from build123d import *

# Parameters (mm, degrees)
SKETCH_1_W          = 41.47467615
SKETCH_1_H          = 18.100023376
EXTRUDE_1_DEPTH     = 2
CUT_EXTRUDE_1_REACH = 26.88
SKETCH_2_R          = 1.4
CUT_EXTRUDE_2_REACH = 26.88


with BuildPart() as part:
    # 草图1 → 凸台-拉伸1 (new body)
    with BuildSketch(Plane.XY):
        with Locations((0, 4.550011688)):
            Rectangle(SKETCH_1_W, SKETCH_1_H)
    extrude(amount=EXTRUDE_1_DEPTH)

    # 草图2 → 切除-拉伸1 (cut, up to next)
    with BuildSketch(Plane.XY.offset(2), mode=Mode.PRIVATE) as cut_extrude_1_sk1:
        with Locations((-18.383061341, -2.4)):
            Circle(SKETCH_2_R)
    cut_extrude_1_tool1 = extrude(cut_extrude_1_sk1.sketch, amount=-CUT_EXTRUDE_1_REACH, mode=Mode.PRIVATE) & part.part
    # 草图2 → 切除-拉伸1 (cut, up to next)
    with BuildSketch(Plane.XY.offset(2), mode=Mode.PRIVATE) as cut_extrude_1_sk2:
        with Locations(Location((18.383061341, -2.4, 0), (0, 0, 180))):
            Circle(SKETCH_2_R)
    cut_extrude_1_tool2 = extrude(cut_extrude_1_sk2.sketch, amount=-CUT_EXTRUDE_1_REACH, mode=Mode.PRIVATE) & part.part
    # 草图2 → 切除-拉伸1 (cut, up to next)
    with BuildSketch(Plane.XY.offset(2), mode=Mode.PRIVATE) as cut_extrude_1_sk3:
        with Locations((18.383061341, 11.500023376)):
            Circle(SKETCH_2_R)
    cut_extrude_1_tool3 = extrude(cut_extrude_1_sk3.sketch, amount=-CUT_EXTRUDE_1_REACH, mode=Mode.PRIVATE) & part.part
    # 草图2 → 切除-拉伸1 (cut, up to next)
    with BuildSketch(Plane.XY.offset(2), mode=Mode.PRIVATE) as cut_extrude_1_sk4:
        with Locations(Location((-18.383061341, 11.500023376, 0), (0, 0, 180))):
            Circle(SKETCH_2_R)
    cut_extrude_1_tool4 = extrude(cut_extrude_1_sk4.sketch, amount=-CUT_EXTRUDE_1_REACH, mode=Mode.PRIVATE) & part.part
    add(cut_extrude_1_tool1.solids().sort_by_distance((-18.383061, -2.4, 2))[0], mode=Mode.SUBTRACT)
    add(cut_extrude_1_tool2.solids().sort_by_distance((18.383061, -2.4, 2))[0], mode=Mode.SUBTRACT)
    add(cut_extrude_1_tool3.solids().sort_by_distance((18.383061, 11.500023, 2))[0], mode=Mode.SUBTRACT)
    add(cut_extrude_1_tool4.solids().sort_by_distance((-18.383061, 11.500023, 2))[0], mode=Mode.SUBTRACT)

    # 草图3 → 切除-拉伸2 (cut, up to next)
    with BuildSketch(Plane(origin=(0, 0, 0), x_dir=(-1, 0, 0), z_dir=(0, 0, -1)), mode=Mode.PRIVATE) as cut_extrude_2_sk1:
        Polygon((-20.737338075, 1.050011688), (-20.437338075, 1.050011688), (-20.237338075, 0.850011688), (-20.237338075, 0.250011688), (-20.437338075, 0.050011688), (-20.737338075, 0.050011688), align=None)
    cut_extrude_2_tool1 = extrude(cut_extrude_2_sk1.sketch, amount=-CUT_EXTRUDE_2_REACH, mode=Mode.PRIVATE) & part.part
    # 草图3 → 切除-拉伸2 (cut, up to next)
    with BuildSketch(Plane(origin=(0, 0, 0), x_dir=(-1, 0, 0), z_dir=(0, 0, -1)), mode=Mode.PRIVATE) as cut_extrude_2_sk2:
        Polygon((-20.737338075, 2.550011688), (-20.437338075, 2.550011688), (-20.237338075, 2.350011688), (-20.237338075, 1.750011688), (-20.437338075, 1.550011688), (-20.737338075, 1.550011688), align=None)
    cut_extrude_2_tool2 = extrude(cut_extrude_2_sk2.sketch, amount=-CUT_EXTRUDE_2_REACH, mode=Mode.PRIVATE) & part.part
    # 草图3 → 切除-拉伸2 (cut, up to next)
    with BuildSketch(Plane(origin=(0, 0, 0), x_dir=(-1, 0, 0), z_dir=(0, 0, -1)), mode=Mode.PRIVATE) as cut_extrude_2_sk3:
        Polygon((-20.737338075, 4.050011688), (-20.437338075, 4.050011688), (-20.237338075, 3.850011688), (-20.237338075, 3.250011688), (-20.437338075, 3.050011688), (-20.737338075, 3.050011688), align=None)
    cut_extrude_2_tool3 = extrude(cut_extrude_2_sk3.sketch, amount=-CUT_EXTRUDE_2_REACH, mode=Mode.PRIVATE) & part.part
    # 草图3 → 切除-拉伸2 (cut, up to next)
    with BuildSketch(Plane(origin=(0, 0, 0), x_dir=(-1, 0, 0), z_dir=(0, 0, -1)), mode=Mode.PRIVATE) as cut_extrude_2_sk4:
        Polygon((-20.737338075, 5.550011688), (-20.437338075, 5.550011688), (-20.237338075, 5.350011688), (-20.237338075, 4.750011688), (-20.437338075, 4.550011688), (-20.737338075, 4.550011688), align=None)
    cut_extrude_2_tool4 = extrude(cut_extrude_2_sk4.sketch, amount=-CUT_EXTRUDE_2_REACH, mode=Mode.PRIVATE) & part.part
    # 草图3 → 切除-拉伸2 (cut, up to next)
    with BuildSketch(Plane(origin=(0, 0, 0), x_dir=(-1, 0, 0), z_dir=(0, 0, -1)), mode=Mode.PRIVATE) as cut_extrude_2_sk5:
        Polygon((-20.737338075, 7.050011688), (-20.437338075, 7.050011688), (-20.237338075, 6.850011688), (-20.237338075, 6.250011688), (-20.437338075, 6.050011688), (-20.737338075, 6.050011688), align=None)
    cut_extrude_2_tool5 = extrude(cut_extrude_2_sk5.sketch, amount=-CUT_EXTRUDE_2_REACH, mode=Mode.PRIVATE) & part.part
    # 草图3 → 切除-拉伸2 (cut, up to next)
    with BuildSketch(Plane(origin=(0, 0, 0), x_dir=(-1, 0, 0), z_dir=(0, 0, -1)), mode=Mode.PRIVATE) as cut_extrude_2_sk6:
        Polygon((-20.737338075, 8.550011688), (-20.437338075, 8.550011688), (-20.237338075, 8.350011688), (-20.237338075, 7.750011688), (-20.437338075, 7.550011688), (-20.737338075, 7.550011688), align=None)
    cut_extrude_2_tool6 = extrude(cut_extrude_2_sk6.sketch, amount=-CUT_EXTRUDE_2_REACH, mode=Mode.PRIVATE) & part.part
    # 草图3 → 切除-拉伸2 (cut, up to next)
    with BuildSketch(Plane(origin=(0, 0, 0), x_dir=(-1, 0, 0), z_dir=(0, 0, -1)), mode=Mode.PRIVATE) as cut_extrude_2_sk7:
        Polygon((-20.737338075, 10.050011688), (-20.437338075, 10.050011688), (-20.237338075, 9.850011688), (-20.237338075, 9.250011688), (-20.437338075, 9.050011688), (-20.737338075, 9.050011688), align=None)
    cut_extrude_2_tool7 = extrude(cut_extrude_2_sk7.sketch, amount=-CUT_EXTRUDE_2_REACH, mode=Mode.PRIVATE) & part.part
    # 草图3 → 切除-拉伸2 (cut, up to next)
    with BuildSketch(Plane(origin=(0, 0, 0), x_dir=(-1, 0, 0), z_dir=(0, 0, -1)), mode=Mode.PRIVATE) as cut_extrude_2_sk8:
        Polygon((20.737338075, 3.050011688), (20.737338075, 4.050011688), (20.437338075, 4.050011688), (20.237338075, 3.850011688), (20.237338075, 3.250011688), (20.437338075, 3.050011688), align=None)
    cut_extrude_2_tool8 = extrude(cut_extrude_2_sk8.sketch, amount=-CUT_EXTRUDE_2_REACH, mode=Mode.PRIVATE) & part.part
    # 草图3 → 切除-拉伸2 (cut, up to next)
    with BuildSketch(Plane(origin=(0, 0, 0), x_dir=(-1, 0, 0), z_dir=(0, 0, -1)), mode=Mode.PRIVATE) as cut_extrude_2_sk9:
        Polygon((20.737338075, 1.550011688), (20.737338075, 2.550011688), (20.437338075, 2.550011688), (20.237338075, 2.350011688), (20.237338075, 1.750011688), (20.437338075, 1.550011688), align=None)
    cut_extrude_2_tool9 = extrude(cut_extrude_2_sk9.sketch, amount=-CUT_EXTRUDE_2_REACH, mode=Mode.PRIVATE) & part.part
    # 草图3 → 切除-拉伸2 (cut, up to next)
    with BuildSketch(Plane(origin=(0, 0, 0), x_dir=(-1, 0, 0), z_dir=(0, 0, -1)), mode=Mode.PRIVATE) as cut_extrude_2_sk10:
        Polygon((20.737338075, 4.550011688), (20.737338075, 5.550011688), (20.437338075, 5.550011688), (20.237338075, 5.350011688), (20.237338075, 4.750011688), (20.437338075, 4.550011688), align=None)
    cut_extrude_2_tool10 = extrude(cut_extrude_2_sk10.sketch, amount=-CUT_EXTRUDE_2_REACH, mode=Mode.PRIVATE) & part.part
    # 草图3 → 切除-拉伸2 (cut, up to next)
    with BuildSketch(Plane(origin=(0, 0, 0), x_dir=(-1, 0, 0), z_dir=(0, 0, -1)), mode=Mode.PRIVATE) as cut_extrude_2_sk11:
        Polygon((20.737338075, 6.050011688), (20.737338075, 7.050011688), (20.437338075, 7.050011688), (20.237338075, 6.850011688), (20.237338075, 6.250011688), (20.437338075, 6.050011688), align=None)
    cut_extrude_2_tool11 = extrude(cut_extrude_2_sk11.sketch, amount=-CUT_EXTRUDE_2_REACH, mode=Mode.PRIVATE) & part.part
    # 草图3 → 切除-拉伸2 (cut, up to next)
    with BuildSketch(Plane(origin=(0, 0, 0), x_dir=(-1, 0, 0), z_dir=(0, 0, -1)), mode=Mode.PRIVATE) as cut_extrude_2_sk12:
        Polygon((20.737338075, 7.550011688), (20.737338075, 8.550011688), (20.437338075, 8.550011688), (20.237338075, 8.350011688), (20.237338075, 7.750011688), (20.437338075, 7.550011688), align=None)
    cut_extrude_2_tool12 = extrude(cut_extrude_2_sk12.sketch, amount=-CUT_EXTRUDE_2_REACH, mode=Mode.PRIVATE) & part.part
    # 草图3 → 切除-拉伸2 (cut, up to next)
    with BuildSketch(Plane(origin=(0, 0, 0), x_dir=(-1, 0, 0), z_dir=(0, 0, -1)), mode=Mode.PRIVATE) as cut_extrude_2_sk13:
        Polygon((20.737338075, 9.050011688), (20.737338075, 10.050011688), (20.437338075, 10.050011688), (20.237338075, 9.850011688), (20.237338075, 9.250011688), (20.437338075, 9.050011688), align=None)
    cut_extrude_2_tool13 = extrude(cut_extrude_2_sk13.sketch, amount=-CUT_EXTRUDE_2_REACH, mode=Mode.PRIVATE) & part.part
    # 草图3 → 切除-拉伸2 (cut, up to next)
    with BuildSketch(Plane(origin=(0, 0, 0), x_dir=(-1, 0, 0), z_dir=(0, 0, -1)), mode=Mode.PRIVATE) as cut_extrude_2_sk14:
        Polygon((20.737338075, 0.050011688), (20.737338075, 1.050011688), (20.437338075, 1.050011688), (20.237338075, 0.850011688), (20.237338075, 0.250011688), (20.437338075, 0.050011688), align=None)
    cut_extrude_2_tool14 = extrude(cut_extrude_2_sk14.sketch, amount=-CUT_EXTRUDE_2_REACH, mode=Mode.PRIVATE) & part.part
    add(cut_extrude_2_tool1.solids().sort_by_distance((20.50328, 0.550012, 0))[0], mode=Mode.SUBTRACT)
    add(cut_extrude_2_tool2.solids().sort_by_distance((20.50328, 2.050012, 0))[0], mode=Mode.SUBTRACT)
    add(cut_extrude_2_tool3.solids().sort_by_distance((20.50328, 3.550012, 0))[0], mode=Mode.SUBTRACT)
    add(cut_extrude_2_tool4.solids().sort_by_distance((20.50328, 5.050012, 0))[0], mode=Mode.SUBTRACT)
    add(cut_extrude_2_tool5.solids().sort_by_distance((20.50328, 6.550012, 0))[0], mode=Mode.SUBTRACT)
    add(cut_extrude_2_tool6.solids().sort_by_distance((20.50328, 8.050012, 0))[0], mode=Mode.SUBTRACT)
    add(cut_extrude_2_tool7.solids().sort_by_distance((20.50328, 9.550012, 0))[0], mode=Mode.SUBTRACT)
    add(cut_extrude_2_tool8.solids().sort_by_distance((-20.50328, 3.550012, 0))[0], mode=Mode.SUBTRACT)
    add(cut_extrude_2_tool9.solids().sort_by_distance((-20.50328, 2.050012, 0))[0], mode=Mode.SUBTRACT)
    add(cut_extrude_2_tool10.solids().sort_by_distance((-20.50328, 5.050012, 0))[0], mode=Mode.SUBTRACT)
    add(cut_extrude_2_tool11.solids().sort_by_distance((-20.50328, 6.550012, 0))[0], mode=Mode.SUBTRACT)
    add(cut_extrude_2_tool12.solids().sort_by_distance((-20.50328, 8.050012, 0))[0], mode=Mode.SUBTRACT)
    add(cut_extrude_2_tool13.solids().sort_by_distance((-20.50328, 9.550012, 0))[0], mode=Mode.SUBTRACT)
    add(cut_extrude_2_tool14.solids().sort_by_distance((-20.50328, 0.550012, 0))[0], mode=Mode.SUBTRACT)


solid = part.part
CAD build for the part. Positions are in the model's coordinates, mm. Give positions to 0.01 mm unless a question says otherwise; leave off trailing zeros. Write each loop counter-clockwise with the first axis right and the second up, starting at its lowest first coordinate (ties: lowest second). Pieces come first, ordered by that corner, then holes. Notation, with made-up numbers: (81.25, -28.5) - (106.25, -28.5) arc R17 cw to (106.25, -6.5) - close; hole circle Ø1 at (55, 12). An arc over 180 degrees is marked (long way). Answer as CSV lines item,"result".
Q1. Pull direction Y, two halves, no side cores. Call faces 1 (the face through (0, 13.6, 1)), 2 (the face through (-19.78, -2.34, 1.01)), 3 (the face through (0, -4.5, 1)), 4 (the face through (0, 5, 0)): released by +Y, released by -Y, zero draft, split by the parting line, or undercut.
Result set:
face 1,"released by +Y"
face 2,"undercut"
face 3,"released by -Y"
face 4,"zero draft"
Q2. Band-saw the part on A-A (y = -2.4). Give the cut face in (x, z).
Result set:
outline,"(-20.74, 0) - (-19.78, 0) - (-19.78, 2) - (-20.74, 2) - close; (-16.98, 0) - (16.98, 0) - (16.98, 2) - (-16.98, 2) - close; (19.78, 0) - (20.74, 0) - (20.74, 2) - (19.78, 2) - close"
Q3. Band-saw the part on C-C (y = 11). Give the cut face in (x, z).
Result set:
outline,"(-20.74, 0) - (-19.69, 0) - (-19.69, 2) - (-20.74, 2) - close; (-17.08, 0) - (17.08, 0) - (17.08, 2) - (-17.08, 2) - close; (19.69, 0) - (20.74, 0) - (20.74, 2) - (19.69, 2) - close"
Q4. Drill centre lines: line 1 (X direction, y = 12, z = 1.6); line 2 (X direction, y = -3, z = 1.45); line 3 (X direction, y = 2, z = 0.6). Where is each one in solid material? Low to high. Write a range as from..to.
Result set:
line 1,"-20.74..-19.69, -17.08..17.08, 19.69..20.74"
line 2,"-20.74..-19.65, -17.12..17.12, 19.65..20.74"
line 3,"-20.24..20.24"
Q5. Band-saw the part on B-B (z = 0.5). State how many separate pieces and enclosed holes the cut face has, and give its area (3 significant figures).
Result set:
separate pieces,"1"
enclosed holes,"4"
area,"720 mm²"
